Autodesk Inventor part; units mm, degrees
ref_plane "YZ Plane" through (0, 0, 0) normal (1, 0, 0) x (0, 1, 0)
ref_plane "XZ Plane" through (0, 0, 0) normal (0, 1, 0) x (-1, 0, 0)
ref_plane "XY Plane" through (0, 0, 0) normal (0, 0, 1) x (1, 0, 0)
sketch "スケッチ1" plane through (0, 0, 0) normal (0, 0, 1) x (1, 0, 0)
  circle A0 centre (0, 0) radius 10
  line L0 (0, 0) -> (12.4, 0)
  line L1 (12.4, 0) -> (12.4, -45)
  line L2 (12.4, -45) -> (-1.6, -45)
  line L3 (-1.6, -45) -> (-1.6, 0)
  circle A1 centre (2.5, -25.5) radius 1.1
  circle A2 centre (2.5, -32) radius 1.7
  circle A3 centre (2.5, -42) radius 1.7
  circle A4 centre (0, 0) radius 5.5
  circle A5 centre (0, 5.5) radius 1.25
  circle A6 centre (0, -5.5) radius 1.25
  circle A7 centre (0, 0) radius 2
  line L4 (0, 0) -> (0, -45)
  line L5 (2.5, -25.5) -> (12.4, -25.5)
  point P0 (7.5, -6.6144)
  point P1 (-1.6, -9.8712)
  point P2 (10, 0)
  dimension "d0" = 20
  dimension "d3" = 12.4
  dimension "d4" = 45
  dimension "d5" = 14
  dimension "d6" = 2.2
  dimension "d7" = 3.4
  dimension "d8" = 3.4
  dimension "d9" = 11
  dimension "d10" = 2.5
  dimension "d11" = 2.5
  dimension "d12" = 4
  dimension "d16" = 2.5
  dimension "d17" = 2.5
  dimension "d18" = 2.5
  dimension "d19" = 9.9
  dimension "d37" = 25.5
extrude "押し出し1" add sketch "スケッチ1" along normal blind 3 contours L0 A4 A5 L3 A0 | L0 L1 L2 L4 A0 | A0 L4 A6 A4 L0 | L3 A4 A6 L4 A0 | A0 L4 L2 L3 | A4 A6 L4 A7 L0 | L0 A7 L3 A4 A5 | L3 A7 L4 A6 A4
fillet "フィレット1" radius 2 1 edges at (-1.6, -9.8712, 1.5)
fillet "フィレット2" radius 4 1 edges at (12.4, 0, 1.5)
fillet "フィレット3" radius 2 1 edges at (10, 0, 1.5)
sketch "スケッチ2" plane through (0, 0, 3) normal (0, 0, 1) x (1, 0, 0)
  line L0 (12.4, -45) -> (12.4, -3.6661)
  line L1 (12.4, -45) -> (12.4, -27)
  line L2 (12.4, -27) -> (-1.6, -27)
  line L3 (-1.6, -11.4473) -> (-1.6, -45)
  line L4 (-1.6, -27) -> (-1.6, -45)
  line L5 (-1.6, -45) -> (12.4, -45)
  line L6 (-1.6, -45) -> (12.4, -45)
  point P0 (0, 0)
  dimension "d22" = 18
extrude "押し出し2" cut sketch "スケッチ2" against normal blind 10
sketch "スケッチ3" plane through (0, 0, 3) normal (0, 0, 1) x (1, 0, 0)
  circle A0 centre (2.5, -25.5) radius 1.1
  line L0 (2.5, -25.5) -> (2.5, -15.5)
  line L1 (2.5, -15.5) -> (10.5, -15.5)
  line L2 (10.5, -15.5) -> (10.5, -27)
  line L3 (-1.6, -27) -> (12.4, -27)
  point P0 (0, 0)
  dimension "d25" = 10
  dimension "d26" = 8
sketch "スケッチ5" plane through (-1.6, -27, 3) normal (0, -1, 0) x (1, 0, 0)
  line L0 (0, -3) -> (0, 0)
  line L1 (0, -1.5) -> (0, -1.3)
  line L2 (0, -1.3) -> (12.1, -1.3)
  line L3 (12.1, -1.3) -> (12.1, -1.7)
  line L4 (12.1, -1.7) -> (0, -1.7)
  line L5 (0, -1.7) -> (0, -1.5)
  point P0 (1.6, -3)
  point P1 (0, -1.7)
  dimension "d32" = 0.2
  dimension "d33" = 12.1
  dimension "d34" = 0.4
extrude "押し出し4" cut sketch "スケッチ5" against normal blind 11.5
sketch "スケッチ6" plane through (-1.6, -27, 3) normal (0, -1, 0) x (1, 0, 0)
  line L0 (12.3614, 0) -> (14, 0)
  line L1 (0, -3) -> (0, 0)
  line L2 (14, 0) -> (0, 0)
  line L3 (0, -1.3) -> (12.1, -1.3)
  line L4 (0, 0) -> (0, -1.3)
  line L5 (12.1, -1.3) -> (12.1, -1.7)
  line L6 (0, -1.3) -> (12.1, -1.3)
  line L7 (12.1, -1.7) -> (0, -1.7)
  line L8 (12.1, -1.3) -> (12.1, -1.7)
  line L9 (12.1, -1.7) -> (0, -1.7)
  line L10 (0, -1.7) -> (0, -3)
  line L11 (0, -3) -> (14, -3)
  line L12 (14, -3) -> (14, 0)
  point P0 (1.6, -3)
extrude "押し出し5" add sketch "スケッチ6" along normal blind 3.5 contours L0 L12 L11 L1 L7 L5 L3 L2
sketch "スケッチ7" plane through (0, 0, 0) normal (0, 0, -1) x (-1, 0, 0)
  line L0 (1.6, -11.4473) -> (1.6, -30.5)
  line L1 (1.6, -30.5) -> (1.6, -15.5)
  line L2 (-10.5, -15.5) -> (1.6, -15.5)
  line L3 (1.6, -15.5) -> (-10.5, -15.5)
  line L4 (-10.5, -15.5) -> (-10.5, -30.5)
  line L5 (-10.5, -30.5) -> (1.6, -30.5)
  point P0 (0, 0)
extrude "押し出し6" cut sketch "スケッチ7" against normal blind 1.5
properties part number "cutter_board_claws_endeffector_8_5_rotary-blade" material "ABS プラスチック"
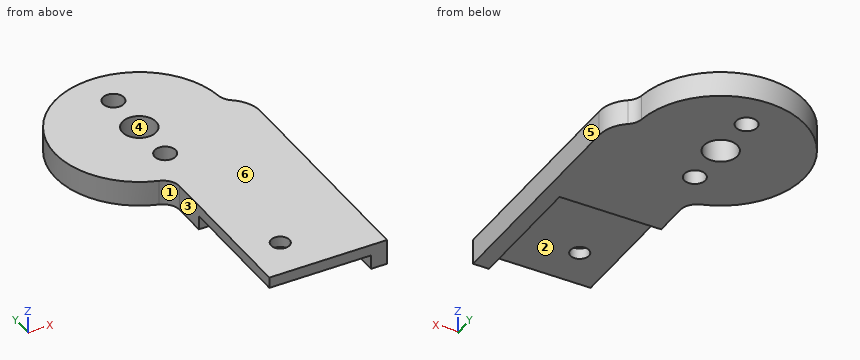
Check sheet for the modelled part. Datum: model origin and axes. Units: mm. Face numbers are marked on the shaded views. A direction names the side the tool comes from. Give positions to 0.01 mm unless a question says otherwise; leave off trailing zeros. Order: outer loops, then holes, each group sorted by start corner. A loop starts at its lowest first (then second) coordinate and runs counter-clockwise, first axis right, second up. Notation, with made-up numbers: (8.25, 11.5) -> (35.25, 11.5) arc R18 ccw to (35.25, 31.5) -> close; hole circle Ø1 at (53, 7.25). An arc over 180 degrees is marked (long way). Use CSV: the item, a comma, the result in double quotes. Start each with the question number.
1) Sectioned sample at B-B, the plane x = 2.5. Record the boundary of the cut face in (y, z), plus the area to 3 significant figures.
2) Set-up check for the marked faces 1 and 2: record each of +Z, -Z, +X, -X, +Y, -Y from which the full face is reachable in a straight line by a thin tool's end or side.
3) Sectioned sample at D-D, the plane y = 5.5. Record the boundary of the cut face in (x, z).
4) Sectioned sample at A-A, the plane y = -25.5. Record the boundary of the cut face in (x, z), plus the area to 3 significant figures.
5) Mould release check, pull along X, two halves, no side actions. Record for the marked faces 3, 4, 5 and 6: released by +X, released by -X, zero draft, split by the parting line, or undercut.
6) Sectioned sample at C-C, the plane z = 2.35. Give the number of separate pieces and of enclosed holes in the cut face, plus the area to 3 significant figures.
7) Material ranges on line 1 (Y direction, x = 0, z = 1.05); line 2 (Y direction, x = 0, z = 1.8); line 3 (X direction, y = -23.5, z = 0.9), recorded low to high. Write a range as from..to.
8) Go/stop test with flat-tipped pins: P1, Ø1, axis at y = -12, z = 1.5, coming from the -X side; P2, Ø0.9, axis at y = -20.5, z = 1, coming from the -X side; P3, Ø6, axis at x = 4.5, y = -24, coming from the -Z side. Record where each tip stops, or that it passes through.
Recorded:
1,outline,"(-30.5, 1.7) -> (-26.6, 1.7) -> (-26.6, 3) -> (-30.5, 3) -> close; (-24.4, 1.7) -> (-15.5, 1.7) -> (-15.5, 0) -> (9.68, 0) -> (9.68, 3) -> (-24.4, 3) -> close"
1,area,"92.2 mm2"
2,face 1,"+Z, -Z, -X, -Y"
2,face 2,"-Z, -X, -Y"
3,outline,"(-8.35, 0) -> (-1.25, 0) -> (-1.25, 3) -> (-8.35, 3) -> close; (1.25, 0) -> (8.35, 0) -> (8.35, 3) -> (1.25, 3) -> close"
4,outline,"(-1.6, 1.7) -> (1.4, 1.7) -> (1.4, 3) -> (-1.6, 3) -> close; (3.6, 1.7) -> (10.5, 1.7) -> (10.5, 0) -> (12.4, 0) -> (12.4, 3) -> (3.6, 3) -> close"
4,area,"18.6 mm2"
5,face 3,"released by -X"
5,face 4,"undercut"
5,face 5,"released by +X"
5,face 6,"zero draft"
6,separate pieces,"1"
6,enclosed holes,"4"
6,area,"619 mm2"
7,line 1,"-15.5..-6.75, -4.25..-2, 2..4.25, 6.75..10"
7,line 2,"-30.5..-6.75, -4.25..-2, 2..4.25, 6.75..10"
7,line 3,"10.5..12.4"
8,P1,"x = -1.6"
8,P2,"x = 10.5"
8,P3,"z = 1.7"
